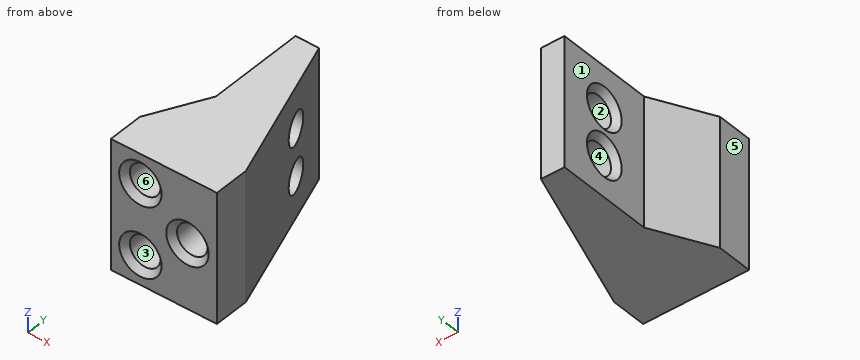
from build123d import *

# Parameters (mm, degrees)
BOSS_EXTRUDE1_DEPTH = 22
SKETCH2_R           = 2.6
CUT_EXTRUDE1_DEPTH  = 14
SKETCH3_R           = 2.6
CUT_EXTRUDE2_DEPTH  = 6
CHAMFER1_SIZE       = 1


with BuildPart() as part:
    # Sketch1 → Boss-Extrude1 (new body)
    with BuildSketch(Plane.XY):
        Polygon((0, 0), (0, 6), (5, 15.65), (5, 32.15), (9, 32.15), (18, 6), (18, 0), align=None)
    extrude(amount=BOSS_EXTRUDE1_DEPTH)

    # Sketch2 → Cut-Extrude1 (cut, through all)
    with BuildSketch(Plane.ZY.offset(-5)):
        with Locations((7, 23.9)):
            Circle(SKETCH2_R)
        with Locations((15, 23.9)):
            Circle(SKETCH2_R)
    extrude(amount=-CUT_EXTRUDE1_DEPTH, mode=Mode.SUBTRACT)

    # Sketch3 → Cut-Extrude2 (cut)
    with BuildSketch(Plane.XZ):
        with Locations((5, 17)):
            Circle(SKETCH3_R)
        with Locations((13, 11)):
            Circle(SKETCH3_R)
        with Locations((5, 5)):
            Circle(SKETCH3_R)
    extrude(amount=-CUT_EXTRUDE2_DEPTH, mode=Mode.SUBTRACT)

    # Chamfer1
    chamfer1_edges = [part.edges().sort_by_distance(p)[0] for p in [
        (5, 23.9, 4.4),
        (5, 23.9, 12.4),
        (2.4, 0, 17),
        (10.4, 0, 11),
        (2.4, 0, 5),
    ]]
    chamfer(chamfer1_edges, length=CHAMFER1_SIZE)


solid = part.part
Part model, mm, in its own coordinate system. Face numbers are marked on the shaded views. A direction names the side the tool comes from. Give positions to 0.01 mm unless a question says otherwise; leave off trailing zeros. Loops run counter-clockwise (first coordinate to the right, second up) from the corner with the lowest first, then second, coordinate; pieces in that order, holes last.
(1) Band-saw the part on B-B (z = 11). Write the cut outline in (x, y), and give its area (3 significant figures).
Return value:
outline: (0, 0) - (9.4, 0) - (10.4, 1) - (10.4, 6) - (15.6, 6) - (15.6, 1) - (16.6, 0) - (18, 0) - (18, 6) - (9, 32.15) - (5, 32.15) - (5, 15.65) - (0, 6) - close
area: 322 mm2
(2) Pull direction X, two halves, no side cores. Call the marked faces 4, 5 and 6: pulls with the +X half, pulls with the -X half, needs draft (parallel to the pull), parting line crosses it, or undercut.
Return value:
face 4: needs draft
face 5: pulls with the -X half
face 6: undercut
(3) Drill centre lines: line 1 along Z through (x, y) = (10, 23.9); line 2 along Z through (x, y) = (5, 3.95); line 3 along Y through (x, z) = (8.75, 15). Where is each one in solid material? Low to high.
Return value:
line 1: z = 0 to 4.4, 9.6 to 12.4, 17.6 to 22
line 2: z = 0 to 2.4, 7.6 to 14.4, 19.6 to 22
line 3: y = 0 to 21.3, 26.5 to 32.15
(4) Band-saw the part on D-D (x = 9.75). Count the separate pieces of the cut face and the enclosed holes in it, and give its area (3 significant figures).
Return value:
separate pieces: 1
enclosed holes: 2
area: 616 mm2
(5) Pin check, flat tips, straight feed: pin 1 (7 mm diameter, centred on x = 5, z = 17, fed in from -Y); pin 2 (3 mm diameter, centred on y = 15.5, z = 3.5, fed in from -X); pin 3 (5.5 mm diameter, centred on x = 13.5, z = 11, fed in from -Y); pin 4 (3 mm diameter, centred on y = 23.9, z = 15, fed in from -X). Stop position of each tip, or through.
Return value:
pin 1: stops at y = 0.1
pin 2: stops at x = 4.15
pin 3: stops at y = 0.35
pin 4: passes through
(6) Band-saw the part on C-C (y = 23.9). Write the cut outline in (x, z), and give its area (3 significant figures).
Return value:
outline: (5, 0) - (11.84, 0) - (11.84, 4.4) - (6, 4.4) - (5, 3.4) - close; (5, 10.6) - (6, 9.6) - (11.84, 9.6) - (11.84, 12.4) - (6, 12.4) - (5, 11.4) - close; (5, 18.6) - (6, 17.6) - (11.84, 17.6) - (11.84, 22) - (5, 22) - close
area: 77.3 mm2
(7) Band-saw the part on A-A (y = 4). Write the cut outline in (x, z), and give its area (3 significant figures).
Return value:
outline: (0, 0) - (18, 0) - (18, 22) - (0, 22) - close; hole circle Ø5.2 at (5, 5); hole circle Ø5.2 at (5, 17); hole circle Ø5.2 at (13, 11)
area: 332 mm2
(8) 3-axis set-ups, long thin cutter, end or side, ignore diameter. For the marked faces 1, 2 and 3: which of +Z, -Z, +X, -X, +Y, -Y reach the whole face in a straight line?
Return value:
face 1: +Z, -Z, -X, +Y
face 2: +X, -X
face 3: -Y
